CAD build for the part. Positions are in the model's coordinates, mm. A direction names the side the tool comes from. Round coordinates to 2 decimals unless told otherwise and drop trailing zeros. Loops run counter-clockwise (first coordinate to the right, second up) from the corner with the lowest first, then second, coordinate; pieces in that order, holes last. Notation, with made-up numbers: M 5.25,78 L 55.25,78 A17 ccw 55.25,83 Z; hole C -18,42 d10. An arc over 180 degrees is marked long. One line per item, written item: value. Start each with the question number.
from build123d import *

# Parameters (mm, degrees)
F0_W          = 43
F0_H          = 43
F1_DEPTH      = 43
F1_DEPTH_BACK = 43
F2_W          = 28
F2_H          = 28
F3_DEPTH      = 71
F4_W          = 28
F4_H          = 28
F5_DEPTH      = 71
F7_DEPTH      = 15
F9_DEPTH      = 100
F10_R         = 1.5
F11_DEPTH     = 2


with BuildPart() as f1:
    # F0 (on Top) → F1 (new body, two sides)
    with BuildSketch(Plane.XY) as f1_sk:
        Polygon((0, 43), (0, 0), (-43, 0), (-43, -43), (0, -43), (43, -43), (43, 0), (43, 43), align=None)
        with Locations((-21.5, 21.5)):
            Rectangle(F0_W, F0_H)
    extrude(amount=F1_DEPTH)
    extrude(f1_sk.sketch, amount=-F1_DEPTH_BACK)

    # F2 (on face) → F3 (cut)
    with BuildSketch(Plane.XY.offset(43)):
        with Locations((-14, 14)):
            Rectangle(F2_W, F2_H)
        Polygon((0, 28), (0, 0), (-28, 0), (-28, -28), (0, -28), (28, -28), (28, 0), (28, 28), align=None)
    extrude(amount=-F3_DEPTH, mode=Mode.SUBTRACT)

    # F4 (on face) → F5 (cut)
    with BuildSketch(Plane.XZ.offset(43)):
        with Locations((-14, 14)):
            Rectangle(F4_W, F4_H)
        Polygon((0, 28), (0, 0), (-28, 0), (-28, -28), (0, -28), (28, -28), (28, 0), (28, 28), align=None)
    extrude(amount=-F5_DEPTH, mode=Mode.SUBTRACT)

    # F6 (on face) → F7 (join)
    with BuildSketch(Plane.YZ.offset(43)):
        Polygon((0, -23), (0, 0), (0, 33), (-43, 33), (-43, -23), align=None)
        Polygon((0, 33), (0, 0), (0, -23), (43, -23), (43, 33), align=None)
    extrude(amount=F7_DEPTH)

    # F8 (on face) → F9 (cut)
    with BuildSketch(Plane.XZ.offset(43)):
        with BuildLine():
            Line((68, 7), (68, 6.5803989155))
            ThreePointArc((68, 6.5803989155), (70.4912121916, 6.8949156836), (73, 7))
            Line((73, 7), (68, 7))
        make_face()
        with BuildLine():
            ThreePointArc((58, 2.9807621135), (47.0192378865, -8), (43, -23))
            Line((43, -23), (58, -23))
            Line((58, -23), (58, 2.9807621135))
        make_face()
    extrude(amount=-F9_DEPTH, mode=Mode.SUBTRACT)

    # F10 (on face) → F11 (join)
    with BuildSketch(Plane.YZ.offset(58)):
        with BuildLine():
            ThreePointArc((-1.5, 15), (-1.0606601718, 13.9393398282), (0, 13.5))
            Line((0, 13.5), (0, 15))
            Line((0, 15), (-1.5, 15))
        make_face()
        with BuildLine():
            Line((-1.5, 15), (0, 15))
            Line((0, 15), (1.5, 15))
            ThreePointArc((1.5, 15), (0, 16.5), (-1.5, 15))
        make_face()
        with BuildLine():
            Line((0, 15), (0, 13.5))
            ThreePointArc((0, 13.5), (1.0606601718, 13.9393398282), (1.5, 15))
            Line((1.5, 15), (0, 15))
        make_face()
        with Locations((-25, 15)):
            Circle(F10_R)
        with BuildLine():
            ThreePointArc((26.5, 15), (25, 16.5), (23.5, 15))
            ThreePointArc((23.5, 15), (25, 13.5), (26.5, 15))
        make_face()
    extrude(amount=F11_DEPTH)


solid = f1.part
(1) Flat gauge pins, fed straight in: P1, Ø9, axis at y = -21, z = 20.5, coming from the +X side; P2, Ø12, axis at x = -11.5, y = 4, coming from the +Z side; P3, Ø22, axis at y = 12.5, z = -35.5, coming from the +X side. Where does each tip first touch, or does it go through?
(2) Which spindle directions (+Z, -Z, +X, -X, +Y, -Y) get a long thin tool onto all of the face, cutting with end or side? Do faces 4 (the cylindrical face through (58.99, -26.5, 15.07)), 5 (the flat face through (28, -8, 7)), 6 (the flat face through (43, -1, 38)). Say none if no direction does.
(3) Slice it at C-C, the plane z = 7.5. List the corners of the cut face in (x, y).
(4) Probe L1, parallel to Y at x = 0, z = 31.5. List the from-to ranges inside material, lowest first.
(5) Mould opens along Z. For faces 1 (the flat face through (60, 25, 15)), 2 (the flat face through (0, -8, -28)), 3 (the flat face through (-1, 29, 43)) say: pulls with the +Z half, pulls with the -Z half, needs draft (parallel to the pull), parting line crosses it, or undercut.
(6) Slice it at D-D, the plane y = -25. List the corners of the cut face in (x, z), and give its area (3 significant figures).
(7) Slice it at B-B, the plane y = 13.5. List the corners of the cut face in (x, z).
(8) Slice it at A-A, the plane x = -15.5. List the corners of the cut face in (y, z).
Check result:
1. P1: stops at x = 58
1. P2: stops at z = -28
1. P3: stops at x = 43
2. face 4: +X
2. face 5: none
2. face 6: +Z, +X, +Y, -Y
3. outline: M -43,-43 L -28,-43 L -28,28 L 28,28 L 28,-43 L 58,-43 L 58,43 L -43,43 Z
4. L1: y = -43 to -28, 28 to 43
5. face 1: needs draft
5. face 2: undercut
5. face 3: pulls with the +Z half
6. outline: M -43,-43 L 43,-43 L 43,-23 A30 cw 58,2.98 L 58,13.5 L 60,13.5 L 60,16.5 L 58,16.5 L 58,33 L 43,33 L 43,43 L 28,43 L 28,-28 L -28,-28 L -28,43 L -43,43 Z
6. area: 3,990 mm^2
7. outline: M -43,-43 L 43,-43 L 43,-23 A30 cw 58,2.98 L 58,33 L 43,33 L 43,43 L 28,43 L 28,-28 L -28,-28 L -28,43 L -43,43 Z
8. outline: M -43,-43 L 43,-43 L 43,43 L 28,43 L 28,-28 L -43,-28 Z; M -43,28 L -28,28 L -28,43 L -43,43 Z
